from build123d import *

# Parameters (mm, degrees)
BOSS_EXTRUDE1_DEPTH            = 10
M5_CLEARANCE_HOLE4_D           = 5.5
M5_CLEARANCE_HOLE4_ON_FACE_2_D = 5.5


with BuildPart() as part:
    # Sketch1 → Boss-Extrude1 (new body)
    with BuildSketch(Plane.XY):
        Polygon((0, 0), (38.1, 0), (38.1, 2), (2, 2), (2, 38.1), (0, 38.1), align=None)
    extrude(amount=BOSS_EXTRUDE1_DEPTH)

    # M5 Clearance Hole4 (through all)
    with Locations(Plane(origin=(2, 12, 5), x_dir=(0, 1, 0), z_dir=(1, 0, 0))):
        with Locations((0, 0), (16.1, 0)):
            Hole(M5_CLEARANCE_HOLE4_D / 2)

    # M5 Clearance Hole4 on face 2 (through all)
    with Locations(Plane(origin=(12, 2, 5), x_dir=(0, 0, 1), z_dir=(0, 1, 0))):
        with Locations((0, 0), (0, 16.1)):
            Hole(M5_CLEARANCE_HOLE4_ON_FACE_2_D / 2)


solid = part.part
CAD build for the part. Positions are in the model's coordinates, mm. A direction names the side the tool comes from. Give positions to 0.01 mm unless a question says otherwise; leave off trailing zeros. Order: outer loops, then holes, each group sorted by start corner. A loop starts at its lowest first (then second) coordinate and runs counter-clockwise, first axis right, second up. Notation, with made-up numbers: (29.5, 85.5) - (79.5, 85.5) arc R19 cw to (79.5, 98.5) - close; hole circle Ø3 at (-13.5, -9.75). An arc over 180 degrees is marked (long way). Answer in a Markdown table with one row per item.
1. Tool access for faces 4 (the flat face through (20, 2, 5)), 5 (the flat face through (19, 0, 5)): list every direction of +Z, -Z, +X, -X, +Y, -Y with a clear straight run to the whole face (end or side of a thin tool).
Data:
| item | result |
|---|---|
| face 4 | +Z, -Z, +X, +Y |
| face 5 | +Z, -Z, +X, -X, -Y |
2. Saw through at A-A, the plane x = 12. Give the cut face in (y, z), plus the area to 3 significant figures.
Data:
| item | result |
|---|---|
| outline | (0, 0) - (2, 0) - (2, 2.25) - (0, 2.25) - close; (0, 7.75) - (2, 7.75) - (2, 10) - (0, 10) - close |
| area | 9.00 mm² |
3. Probe probe 1 along X at (y, z) = (0.95, 5); probe 2 along Z at (x, y) = (1, 12); probe 3 along X at (y, z) = (29, 9.75). List the from-to ranges inside material, lowest first. Write a range as [from, to].
Data:
| item | result |
|---|---|
| probe 1 | x = [0, 9.25], [14.75, 25.35], [30.85, 38.1] |
| probe 2 | z = [0, 2.25], [7.75, 10] |
| probe 3 | x = [0, 2] |
4. Flat gauge pins, fed straight in: pin 1 (1 mm diameter, centred on y = 8, z = 2.5, fed in from +X); pin 2 (3 mm diameter, centred on x = 5, z = 6.5, fed in from +Y); pin 3 (1 mm diameter, centred on y = 8.5, z = 8.5, fed in from -X). Where does each tip first touch, or does it go through?
Data:
| item | result |
|---|---|
| pin 1 | stops at x = 2 |
| pin 2 | stops at y = 2 |
| pin 3 | stops at x = 0 |
5. Saw through at D-D, the plane z = 9.25. Give the cut face in (x, y).
Data:
| item | result |
|---|---|
| outline | (0, 0) - (38.1, 0) - (38.1, 2) - (2, 2) - (2, 38.1) - (0, 38.1) - close |
6. Pull direction X, two halves, no side cores. Call faces 1 (the cylindrical face through (12.83, 0.99, 2.38)), 2 (the flat face through (38.1, 1, 5)), 3 (the flat face through (1, 11, 10)): pulls with the +X half, pulls with the -X half, needs draft (parallel to the pull), parting line crosses it, or undercut.
Data:
| item | result |
|---|---|
| face 1 | undercut |
| face 2 | pulls with the +X half |
| face 3 | needs draft |
7. Saw through at B-B, the plane z = 5. Give the cut face in (x, y).
Data:
| item | result |
|---|---|
| outline | (0, 0) - (9.25, 0) - (9.25, 2) - (2, 2) - (2, 9.25) - (0, 9.25) - close; (0, 14.75) - (2, 14.75) - (2, 25.35) - (0, 25.35) - close; (0, 30.85) - (2, 30.85) - (2, 38.1) - (0, 38.1) - close; (14.75, 0) - (25.35, 0) - (25.35, 2) - (14.75, 2) - close; (30.85, 0) - (38.1, 0) - (38.1, 2) - (30.85, 2) - close |
